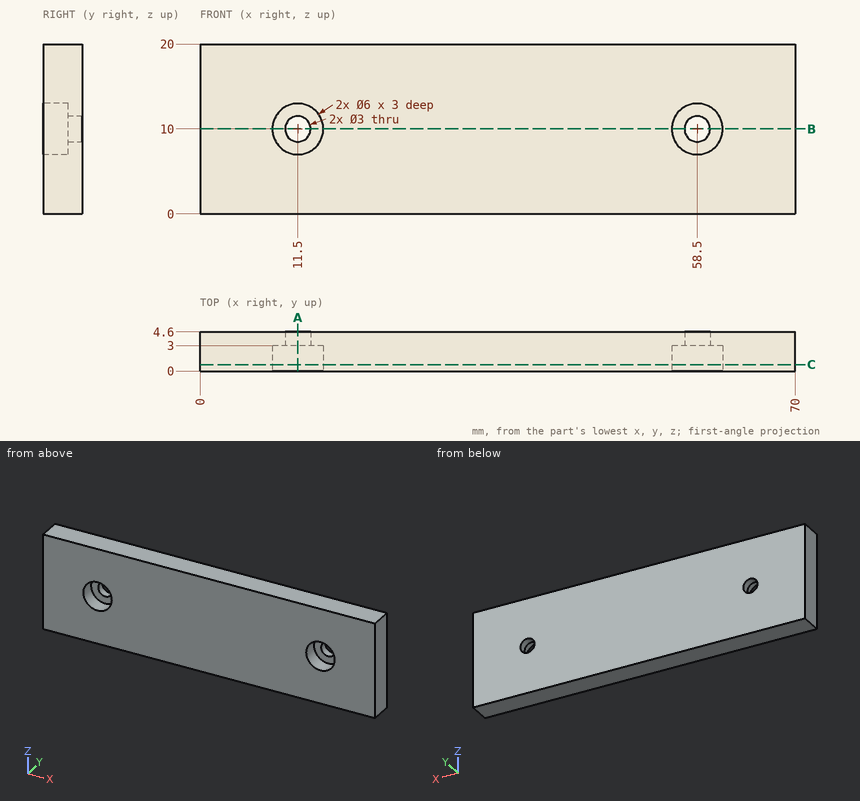
Here's the drawing with two shaded views (mm, measured from the low corner). I have some questions. Give positions to 0.01 mm unless a question says otherwise; leave off trailing zeros. Loops run counter-clockwise (first coordinate to the right, second up) from the corner with the lowest first, then second, coordinate; pieces in that order, holes last. Notation, with made-up numbers: (22.5, 51.5) - (29.5, 51.5) arc R8 ccw to (29.5, 63.5) - close; hole circle Ø7 at (16, 27.25). An arc over 180 degrees is marked (long way). One line per item, written item: value.
(1) I need wall thicknesses on line 1 along X through (y, z) = (0.55, 10.25); line 2 along X through (y, z) = (3.75, 10); line 3 along Z through (x, y) = (58.5, 4.2). Which ranges of each line are inside material? Lowest first, please.
Verdict:
line 1: 0 to 8.51, 14.49 to 55.51, 61.49 to 70
line 2: 0 to 10, 13 to 57, 60 to 70
line 3: 0 to 8.5, 11.5 to 20
(2) If we section it at C-C, the plane y = 0.75: List the corners of the cut face in (x, z) for me, plus the area to 3 significant figures.
Verdict:
outline: (0, 0) - (70, 0) - (70, 20) - (0, 20) - close; hole circle Ø6 at (11.5, 10); hole circle Ø6 at (58.5, 10)
area: 1,340 mm^2
(3) If we section it at B-B, the plane z = 10: List the corners of the cut face in (x, y) for me, plus the area to 3 significant figures.
Verdict:
outline: (0, 0) - (8.5, 0) - (8.5, 3) - (10, 3) - (10, 4.6) - (0, 4.6) - close; (13, 3) - (14.5, 3) - (14.5, 0) - (55.5, 0) - (55.5, 3) - (57, 3) - (57, 4.6) - (13, 4.6) - close; (60, 3) - (61.5, 3) - (61.5, 0) - (70, 0) - (70, 4.6) - (60, 4.6) - close
area: 276 mm^2
(4) I'm going to push flat-ended pins straight in: pin 1 (2.5 mm diameter, centred on x = 58.5, z = 10, fed in from +Y); pin 2 (3.5 mm diameter, centred on x = 11.5, z = 10, fed in from -Y). Where does each tip first touch, or does it pass through?
Verdict:
pin 1: through
pin 2: y = 3
(5) If we section it at A-A, the plane x = 11.5: List the corners of the cut face in (y, z) for me.
Verdict:
outline: (0, 0) - (4.6, 0) - (4.6, 8.5) - (3, 8.5) - (3, 7) - (0, 7) - close; (0, 13) - (3, 13) - (3, 11.5) - (4.6, 11.5) - (4.6, 20) - (0, 20) - close
